Autodesk Inventor part; units mm, degrees
ref_plane "Work Plane1" through (11, 0, 4) normal (1, 0, 0) x (0, 1, 0)
ref_plane "Work Plane2" through (0, 0, -7) normal (0, 0, -1) x (-1, 0, 0)
ref_plane "YZ Plane" through (0, 0, 0) normal (1, 0, 0) x (0, 1, 0)
sketch "Sketch1" plane through (0, 0, 0) normal (0, 0, 1) x (1, 0, 0)
  circle A0 centre (0, 0) radius 2.5
  circle A1 centre (20, 0) radius 2.5
  line L0 (7, 10) -> (20, 10)
  line L1 (7, -10) -> (20, -10)
  arc A2 (20, -10) -> (20, 10) centre (20, 0) ccw
  line L2 (7, 10) -> (7, 8)
  line L3 (7, -10) -> (7, -8)
  line L4 (7, 8) -> (0, 8)
  line L5 (7, -8) -> (0, -8)
  arc A3 (0, 8) -> (0, -8) centre (0, 0) ccw
  dimension "d0" = 5
  dimension "d1" = 20
  dimension "d2" = 10
  dimension "d3" = 2
  dimension "d4" = 13
extrude "Extrusion1" add sketch "Sketch1" along normal blind 4
sketch "Sketch2" plane through (0, 0, 4) normal (0, 0, 1) x (1, 0, 0)
  circle A0 centre (0, 0) radius 2.5
  line L0 (7, 8) -> (0, 8)
  arc A1 (0, 8) -> (0, -8) centre (0, 0) ccw
  line L1 (0, -8) -> (7, -8)
  line L2 (7, -10) -> (20, -10)
  line L3 (7, 8) -> (7, -8)
  line L4 (7, -8) -> (0, -8)
  line L5 (7, 8) -> (0, 8)
  arc A2 (0, 8) -> (0, -8) centre (0, 0) ccw
extrude "Extrusion2" cut sketch "Sketch2" against normal blind 2
sketch "Sketch3" plane through (0, 0, 0) normal (0, 0, -1) x (-1, 0, 0)
  circle A0 centre (-20, 0) radius 2.5
  circle A1 centre (0, 0) radius 2.5
  line L0 (-7, 10) -> (-20, 10)
  arc A2 (-20, 10) -> (-20, -10) centre (-20, 0) ccw
  line L1 (-20, -10) -> (-7, -10)
  line L2 (-7, 8) -> (-7, 10)
  line L3 (-19, 10) -> (-19, 8)
  line L4 (-19, 8) -> (-11, 8)
  line L5 (-11, 8) -> (-11, -8)
  line L6 (-11, -8) -> (-19, -8)
  line L7 (-19, -8) -> (-19, -10)
  point P0 (-7, -8)
  dimension "d9" = 1
  dimension "d10" = 11
extrude "Extrusion3" cut sketch "Sketch3" against normal blind 2 contours L3 L4 L5 L6 L7 L1 A2 L0
sketch "Sketch4" plane through (0, 0, 4) normal (0, 0, 1) x (1, 0, 0)
  line L0 (7, 10) -> (7, -10)
  circle A0 centre (0, 0) radius 2.5
  arc A1 (7, -8.485281) -> (7, 8.485281) centre (0, 0) ccw
  dimension "d15" = 11
extrude "Extrusion4" cut sketch "Sketch4" against normal blind 2 contours A1 L0
sketch "Sketch5" plane through (0, 0, 0) normal (0, 0, -1) x (-1, 0, 0)
  line L0 (0, 8) -> (-7, 8)
  line L1 (-7, 10) -> (0, 10)
  line L2 (0, 10) -> (0, 8)
  line L3 (0, 8) -> (-7, 8)
  line L4 (-7, 8) -> (-7, 10)
  arc A0 (0, -8) -> (0, 8) centre (0, 0) ccw
extrude "Extrusion5" add sketch "Sketch5" against normal blind 2
sketch "Sketch6" plane through (0, 0, 0) normal (0, 0, -1) x (-1, 0, 0)
  line L0 (0, 10) -> (-19, 10)
  line L1 (-19, 8) -> (-20, 8)
  line L2 (-20, 8) -> (-20, 10)
  line L3 (-20, 10) -> (-19, 10)
  line L4 (-19, 10) -> (-19, 8)
  circle A0 centre (-20, 0) radius 2.5
extrude "Extrusion6" add sketch "Sketch6" against normal blind 2 contours L1 L2 L3 L4
sketch "Sketch7" plane through (0, 0, 0) normal (0, 0, -1) x (-1, 0, 0)
  line L0 (-19, -8) -> (-19, -10)
  line L1 (-11, -8) -> (-19, -8)
  line L2 (-17.400642, -8) -> (-19, -9.162001)
  line L3 (-17.400642, -8) -> (-26.805206, 4.944272) construction
  line L4 (-26.805206, 4.944272) -> (-28.404564, 3.782271) construction
  line L5 (-28.404564, 3.782271) -> (-19, -9.162001) construction
  circle A0 centre (-20, 0) radius 2.5
  line L6 (-17.400642, -8) -> (-19, -8)
  line L7 (-19, -8) -> (-19, -9.162001)
  dimension "d21" = 16
  dimension "d22" = 8
  dimension "d23" = 36
extrude "Extrusion7" cut sketch "Sketch7" against normal blind 2 contours L1 L2 L0
sketch "Sketch9" plane through (0, 0, 2) normal (0, 0, 1) x (1, 0, 0)
  circle A0 centre (0, 0) radius 2.5
  arc A1 (11, 0) -> (7, 8.485281) centre (0, 0) ccw
  circle A2 centre (0, 0) radius 2.5
extrude "Extrusion8" add sketch "Sketch9" along normal mid plane 4
fillet "Fillet1" radius 0.5 1 edges at (-2.5, 0, 4)
sketch "Sketch10" plane through (0, 0, 0) normal (0, 0, -1) x (-1, 0, 0)
  arc A0 (0, -8) -> (0, 8) centre (0, 0) ccw
  line L0 (0, 10) -> (-20, 10)
  line L1 (4.702282, 6.472136) -> (11.174418, 1.769854)
  line L2 (11.174418, 1.769854) -> (6.472136, -4.702282)
  dimension "d30" = 144
extrude "Extrusion9" add sketch "Sketch10" against normal blind 2
fillet "Fillet2" radius 6 1 edges at (-11.1744, 1.7699, 1)
ref_plane "Work Plane1" through (11, 0, 4) normal (1, 0, 0) x (0, 1, 0)
split "Split1" plane through (11, 0, 4) removes the side toward (1, 0, 0)
sketch "Sketch11" plane through (11, -10, 0) normal (1, 0, 0) x (0, 0, -1)
  line L0 (0, 20) -> (0, 0)
  line L1 (-4, 20) -> (0, 20)
  line L2 (-4, 10) -> (-4, 20)
  line L3 (-4, 0) -> (-4, 10)
  line L4 (0, 0) -> (-4, 0)
  point P0 (0, 10)
extrude "Extrusion10" add sketch "Sketch11" along normal blind 1
ref_plane "Work Plane2" through (0, 0, -7) normal (0, 0, -1) x (-1, 0, 0)
mirror "Mirror1" about plane through (0, 0, -7) normal (0, 0, -1)
sketch "Sketch12" plane through (0, 0, 0) normal (0, 0, -1) x (-1, 0, 0)
  line L0 (-12, -10) -> (-7, -10)
  line L1 (-7, -10) -> (-7, -8)
  arc A0 (4.702282, 6.472136) -> (0, 8) centre (0, 0) ccw
  line L2 (0, 8) -> (0, 10)
  line L3 (0, 10) -> (-12, 10)
  line L4 (-12, -10) -> (-12, 10)
  line L5 (0, 8) -> (-12, 8)
  line L6 (-7, -8) -> (-12, -8)
extrude "Extrusion11" add sketch "Sketch12" along normal blind 14
sketch "Sketch13" plane through (12, -10, 0) normal (1, 0, 0) x (0, 0, -1)
  line L0 (0, 18) -> (14, 18)
  line L1 (0, 2) -> (14, 2)
  line L2 (-4, 0) -> (18, 0)
  line L3 (18, 20) -> (18, 0)
  line L4 (-4, 20) -> (18, 20)
  line L5 (-4, 20) -> (-4, 0)
  line L6 (-2, 18) -> (16, 18)
  line L7 (16, 18) -> (16, 2)
  line L8 (16, 2) -> (-2, 2)
  line L9 (-2, 2) -> (-2, 18)
  point P0 (0, 10)
  dimension "d39" = 2
  dimension "d40" = 2
extrude "Extrusion12" add sketch "Sketch13" along normal blind 20
sketch "Sketch17" plane through (0, 0, 4) normal (0, 0, 1) x (1, 0, 0)
  line L0 (7, -10) -> (32, -10)
  line L1 (32, 10) -> (32, -10)
  line L2 (32, 6) -> (12, -10)
  dimension "d73" = 4
  dimension "d74" = 20
extrude "Extrusion16" cut sketch "Sketch17" against normal blind 22
sketch "Sketch18" plane through (0, 8, 0) normal (0, -1, 0) x (1, 0, 0)
  line L0 (12, -16) -> (32, -16)
  line L1 (32, 2) -> (32, -16)
  line L2 (12, 2) -> (32, 2)
  line L3 (15, -1) -> (29, -1) construction
  line L4 (29, -1) -> (29, -13) construction
  line L5 (29, -13) -> (15, -13) construction
  line L6 (15, -13) -> (15, -1) construction
  circle A0 centre (15, -13) radius 1.7
  circle A1 centre (15, -1) radius 1.7
  circle A2 centre (29, -1) radius 1.7
  circle A3 centre (29, -13) radius 1.7
  line L7 (20, -1) -> (24, -1)
  line L8 (28, -5) -> (28, -9)
  line L9 (24, -13) -> (20, -13)
  line L10 (16, -9) -> (16, -5)
  line L11 (16, -9) -> (20, -13)
  line L12 (24, -13) -> (28, -9)
  line L13 (28, -5) -> (24, -1)
  line L14 (20, -1) -> (16, -5)
  point P0 (16, -7)
  point P1 (15, -7)
  dimension "d77" = 3.4
  dimension "d78" = 45
  dimension "d79" = 4
  dimension "d80" = 3
  dimension "d81" = 3
  dimension "d82" = 3
  dimension "d83" = 14
  dimension "d84" = 1
  dimension "d85" = 1
extrude "Extrusion17" cut sketch "Sketch18" against normal through all
properties part number "y_axis_cable_mount_b" material "ABS Plastic"
Read the model definition and answer for the solid it produces. Units are mm, in the model's axes. A direction names the side the tool comes from. Round coordinates to 2 decimals unless told otherwise and drop trailing zeros. Write each loop counter-clockwise with the first axis right and the second up, starting at its lowest first coordinate (ties: lowest second). Pieces come first, ordered by that corner, then holes.
Q1. Find section B-B on z = -8.5. Determine the outline of the cut face in (x, y).
Values:
outline: (0, 8) - (16, 8) - (16, 10) - (0, 10) - close; (7, -10) - (12, -10) - (14.5, -8) - (7, -8) - close; (28, 8) - (32, 8) - (32, 10) - (28, 10) - close
Q2. A tool of negligible diameter and unlimited length cuts with its end or side. For faces 1 (the face through (16, 9, -7)), 2 (the face through (1, 0, 0)), 3 (the face through (4, -8, 1)), 4 (the face through (7, 9, -17)), 5 (the face through (12, 0, -15)), from which of +Z, -Z, +X, -X, +Y, -Y can it reach the whole face along a straight path? Write none if from no direction.
Values:
face 1: +Y, -Y
face 2: +X, -X
face 3: +Z, -Z, -X, -Y
face 4: -Z, -X, +Y, -Y
face 5: +X
Q3. Straight lines are drawn through the part: line 1 (Z direction, x = 29, y = 9.3); line 2 (Y direction, x = 12, z = -8.25); line 3 (Z direction, x = 8, y = 1.25). For each, find the intervals that lie inside material, in ascending order.
Values:
line 1: z = -18 to -14.7, -11.3 to -2.7, 0.7 to 4
line 2: y = -10 to -8, 8 to 10
line 3: z = -16 to -14, 0 to 2
Q4. Flat-ended cylindrical pins translate along their axes: P1, Ø3, axis at x = 4.5, y = 3, coming from the -Z side; P2, Ø1.2, axis at y = 9, z = -17.5, coming from the -X side; P3, Ø1, axis at x = 3, z = -14.5, coming from the -Y side; P4, Ø5, axis at y = -3.5, z = -8, coming from the -X side. Find the tip coordinate at first contact, or state that the pin passes through.
Values:
P1: stops at z = -16
P2: stops at x = 7
P3: stops at y = -8
P4: passes through
Q5. Find section A-A on x = 21. Determine the outline of the cut face in (y, z), and give its area (3 significant figures).
Values:
outline: (-2.8, -18) - (10, -18) - (10, -13) - (8, -13) - (8, -16) - (-2.8, -16) - close; (-2.8, 2) - (8, 2) - (8, -1) - (10, -1) - (10, 4) - (-2.8, 4) - close
area: 63.2 mm2
Q6. The mould has two halves that part along Z. Classify faces 6 (the face through (32, 8.5, -6.8)), 7 (the face through (12, 0, 1)), 8 (the face through (3, 1, -16)): released by +Z, released by -Z, zero draft, split by the parting line, or undercut.
Values:
face 6: zero draft
face 7: undercut
face 8: released by -Z
Q7. Find section D-D on z = 2.75. Determine the outline of the cut face in (x, y), and give its area (3 significant figures).
Values:
outline: circle Ø5 at (0, 0); (7, -10) - (12, -10) - (32, 6) - (32, 10) - (7, 10) - (7, 8.49) arc R11 cw to (7, -8.49) - close
area: 312 mm2
Q8. Find section C-C on x = 15. Determine the outline of the cut face in (y, z).
Values:
outline: (-7.6, -18) - (10, -18) - (10, -14.7) - (8, -14.7) - (8, -16) - (-7.6, -16) - close; (-7.6, 2) - (8, 2) - (8, 0.7) - (10, 0.7) - (10, 4) - (-7.6, 4) - close; (8, -11.3) - (10, -11.3) - (10, -2.7) - (8, -2.7) - close
